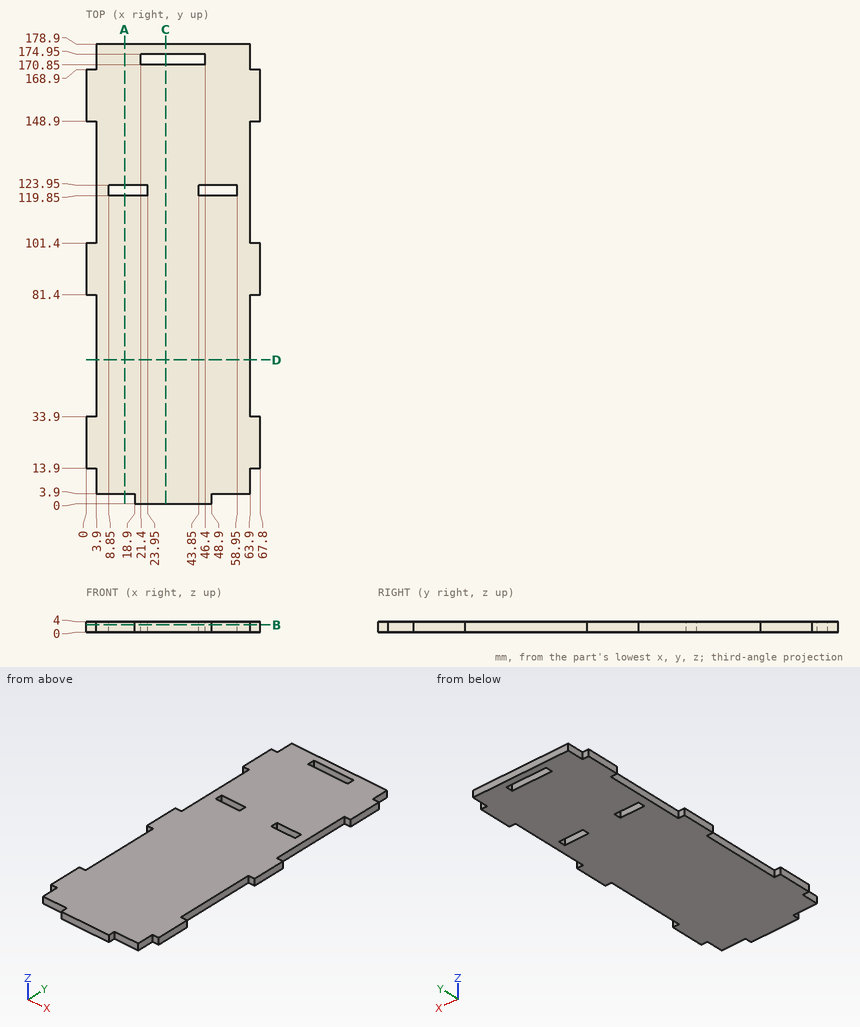
The drawing under review shows one solid part. Ordinate dimensions are in mm from its lowest x, y, z. Give positions to 0.01 mm unless a question says otherwise; leave off trailing zeros. Order: outer loops, then holes, each group sorted by start corner. A loop starts at its lowest first (then second) coordinate and runs counter-clockwise, first axis right, second up. Notation, with made-up numbers: M -27.75,58.5 L -8.75,58.5 A10 cw -8.75,66.5 Z; hole C 37,49.25 d1. An arc over 180 degrees is marked long. One line per question, with ' | ' between items. Start each with the question number.
Q1. We need section B-B (z = 2.8). State how many separate pieces and enclosed holes the cut face has, plus the area to 3 significant figures.
Q2. For pin 1 Ø1.2 at (y, z) = (56, 2.5) entering from +X; pin 2 Ø1.2 at (x, z) = (66, 2.5) entering from +Y; pin 3 Ø1.2 at (y, z) = (9.5, 2.5) entering from -X; pin 4 Ø2 at (x, z) = (38, 2.5) entering from -Y, all flat-tipped, find the tip position at first contact; note any pin that passes through.
Q3. We need section A-A (x = 15). Write out the cut boundary in (y, z).
Q4. For L1, parallel to Y at x = 48, z = 1; L2, parallel to Y at x = 52.5, z = 2; L3, parallel to X at y = 12, z = 3.15, list the stretches that pass through material, from the lowest coordinate up. Write a range as [from, to].
Q5. We need section D-D (y = 56). Write out the cut boundary in (x, z).
Q6. We need section C-C (x = 31). Write out the cut boundary in (y, z), plus the area to 3 significant figures.
Returned:
1) separate pieces: 1 | enclosed holes: 3 | area: 10,900 mm2
2) pin 1: x = 63.9 | pin 2: y = 168.9 | pin 3: x = 3.9 | pin 4: y = 0
3) outline: M 3.9,0 L 119.85,0 L 119.85,4 L 3.9,4 Z; M 123.95,0 L 178.9,0 L 178.9,4 L 123.95,4 Z
4) L1: [0, 119.85], [123.95, 178.9] | L2: [3.9, 119.85], [123.95, 178.9] | L3: [3.9, 63.9]
5) outline: M 3.9,0 L 63.9,0 L 63.9,4 L 3.9,4 Z
6) outline: M 0,0 L 170.85,0 L 170.85,4 L 0,4 Z; M 174.95,0 L 178.9,0 L 178.9,4 L 174.95,4 Z | area: 699 mm2
